from build123d import *

# Parameters (mm, degrees)
BOSS_EXTRUDE1_DEPTH = 5
CUT_EXTRUDE1_DEPTH  = 86.941840799
BOSS_EXTRUDE2_DEPTH = 5
SKETCH7_R           = 4.1
CUT_EXTRUDE2_DEPTH  = 86.941840799
FILLET1_R           = 1


with BuildPart() as part:
    # Sketch1 → Boss-Extrude1 (new body)
    with BuildSketch(Plane(origin=(0, 0, 0), x_dir=(0, 0, -1), z_dir=(1, 0, 0))):
        Polygon((0, 0), (0, -81), (14.142135624, -66.857864376), (28.284271247, -81), (28.284271247, 0), (14.142135624, -14.142135624), align=None)
    extrude(amount=BOSS_EXTRUDE1_DEPTH)

    # Sketch2 → Cut-Extrude1 (cut, through all)
    with BuildSketch(Plane(origin=(5, 0, 0), x_dir=(0, 0, -1), z_dir=(1, 0, 0))):
        Polygon((4, -71.343145751), (12.142135624, -63.201010127), (12.142135624, -17.798989873), (4, -9.656854249), align=None)
        Polygon((16.142135624, -17.798989873), (16.142135624, -63.201010127), (24.284271247, -71.343145751), (24.284271247, -9.656854249), align=None)
    extrude(amount=-CUT_EXTRUDE1_DEPTH, mode=Mode.SUBTRACT)

    # Sketch6 → Boss-Extrude2 (add, through all)
    with BuildSketch(Plane(origin=(5, 0, 0), x_dir=(0, 0, -1), z_dir=(1, 0, 0))):
        with BuildLine():
            Line((20.850339556, -42.5), (16.142135624, -42.5))
            Line((16.142135624, -42.5), (16.142135624, -47.208203932))
            ThreePointArc((16.142135624, -47.208203932), (19.091883092, -45.449747468), (20.850339556, -42.5))
        make_face()
        with BuildLine():
            Line((20.850339556, -38.5), (16.142135624, -38.5))
            Line((16.142135624, -38.5), (16.142135624, -42.5))
            Line((16.142135624, -42.5), (20.850339556, -42.5))
            ThreePointArc((20.850339556, -42.5), (21.068802482, -41.510587075), (21.142135624, -40.5))
            ThreePointArc((21.142135624, -40.5), (21.068802482, -39.489412925), (20.850339556, -38.5))
        make_face()
        with BuildLine():
            Line((16.142135624, -33.791796068), (16.142135624, -38.5))
            Line((16.142135624, -38.5), (20.850339556, -38.5))
            ThreePointArc((20.850339556, -38.5), (19.091883092, -35.550252532), (16.142135624, -33.791796068))
        make_face()
        with BuildLine():
            ThreePointArc((12.142135624, -33.791796068), (9.192388155, -35.550252532), (7.433931691, -38.5))
            Line((7.433931691, -38.5), (12.142135624, -38.5))
            Line((12.142135624, -38.5), (12.142135624, -33.791796068))
        make_face()
        with BuildLine():
            Line((12.142135624, -42.5), (7.433931691, -42.5))
            ThreePointArc((7.433931691, -42.5), (9.192388155, -45.449747468), (12.142135624, -47.208203932))
            Line((12.142135624, -47.208203932), (12.142135624, -42.5))
        make_face()
        with BuildLine():
            Line((12.142135624, -38.5), (7.433931691, -38.5))
            ThreePointArc((7.433931691, -38.5), (7.142135624, -40.5), (7.433931691, -42.5))
            Line((7.433931691, -42.5), (12.142135624, -42.5))
            Line((12.142135624, -42.5), (12.142135624, -38.5))
        make_face()
        with BuildLine():
            Line((7.433931691, -38.5), (4, -38.5))
            Line((4, -38.5), (4, -42.5))
            Line((4, -42.5), (7.433931691, -42.5))
            ThreePointArc((7.433931691, -42.5), (7.142135624, -40.5), (7.433931691, -38.5))
        make_face()
        with BuildLine():
            Line((24.284271247, -38.5), (20.850339556, -38.5))
            ThreePointArc((20.850339556, -38.5), (21.068802482, -39.489412925), (21.142135624, -40.5))
            ThreePointArc((21.142135624, -40.5), (21.068802482, -41.510587075), (20.850339556, -42.5))
            Line((20.850339556, -42.5), (24.284271247, -42.5))
            Line((24.284271247, -42.5), (24.284271247, -38.5))
        make_face()
    extrude(amount=-BOSS_EXTRUDE2_DEPTH)

    # Sketch7 → Cut-Extrude2 (cut, through all)
    with BuildSketch(Plane(origin=(5, 0, 0), x_dir=(0, 0, -1), z_dir=(1, 0, 0))):
        with Locations((14.142135624, -40.5)):
            Circle(SKETCH7_R)
    extrude(amount=-CUT_EXTRUDE2_DEPTH, mode=Mode.SUBTRACT)

    # Fillet1
    fillet1_edges = [part.edges().sort_by_distance(p)[0] for p in [
        (2.5, 0, 0),
        (2.5, 0, -28.284271247),
        (2.5, -81, -28.284271247),
        (2.5, -81, 0),
        (2.5, -17.798989873, -12.142135624),
        (2.5, -63.201010127, -12.142135624),
        (2.5, -71.343145751, -4),
        (2.5, -9.656854249, -4),
        (2.5, -9.656854249, -24.284271247),
        (2.5, -71.343145751, -24.284271247),
        (2.5, -63.201010127, -16.142135624),
        (2.5, -17.798989873, -16.142135624),
    ]]
    fillet(fillet1_edges, radius=FILLET1_R)


solid = part.part
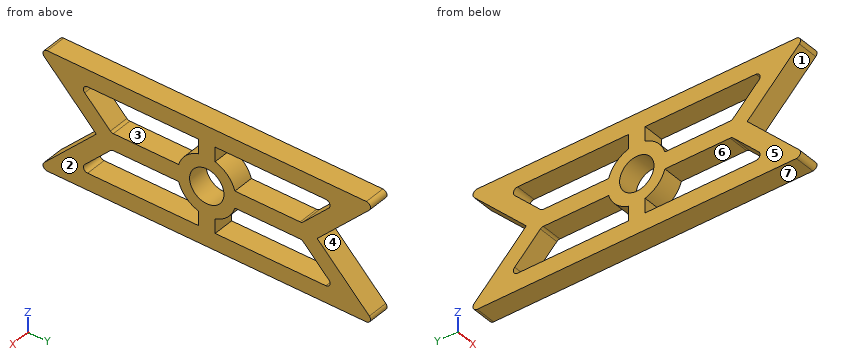
Design review of the part built by this model. Coordinates are the model's own, in mm. Face numbers are marked on the shaded views. A direction names the side the tool comes from. Give positions to 0.01 mm unless a question says otherwise; leave off trailing zeros. Loops run counter-clockwise (first coordinate to the right, second up) from the corner with the lowest first, then second, coordinate; pieces in that order, holes last. Notation, with made-up numbers: (78.25, -3) - (126.25, -3) arc R25 cw to (126.25, 29) - close; hole circle Ø11 at (-39, -14). An arc over 180 degrees is marked (long way). Use CSV: the item, a comma, the result in double quotes. Start each with the question number.
1. Add section B-B (y = -40.5). State the section outline as (x, z) points, plus the area to 3 significant figures.
2. Add section C-C (z = -17.5). State the section outline as (x, y) points.
3. Draft analysis for pull direction Z (two halves, no side actions). For the marked faces 5, 6 and 7, state which applies: released by +Z, released by -Z, zero draft, split by the parting line, or undercut.
4. Machinability: for the marked faces 1, 2, 3 and 4, which of the approach directions +Z, -Z, +X, -X, +Y, -Y give a long, thin tool a straight path to every point of the face, cutting with its end or side? Answer none if there is none.
5. Add section A-A (y = -58). State the section outline as (x, z) points, plus the area to 3 significant figures.
6. Wall thickness on L1, parallel to Z at x = 4.1, y = -26; L2, parallel to Y at x = 1.35, z = -11.5; L3, parallel to Y at x = 1.6, z = -19.5: over which ranges is each line inside the solid? List them lowest first.
7. Insertion check: P1, Ø1.5, axis at x = 2.5, z = -7, coming from the +Y side; P2, Ø2.5, axis at x = 2, z = -5.5, coming from the -Y side; P3, Ø1.7, axis at x = 3.5, z = -6, coming from the +Y side; P4, Ø4, axis at y = -26.5, z = -18.5, coming from the -X side. Each pin has a flat end and moves straight along its axis. Give the tip position at first contact, or say it passes through.
8. Add section D-D (x = 1.55). Count the separate pieces of the cut face and the enclosed holes in it, plus the area to 3 significant figures.
Results found:
1,outline,"(0, -28.28) - (5, -28.28) - (5, -18.24) - (0, -18.24) - close; (0, -10.04) - (5, -10.04) - (5, 0) - (0, 0) - close"
1,area,"100 mm²"
2,outline,"(0, -70.22) - (5, -70.22) - (5, -64.56) - (0, -64.56) - close; (0, -46.64) - (5, -46.64) - (5, -42.85) - (0, -42.85) - close; (0, -38.15) - (5, -38.15) - (5, -34.36) - (0, -34.36) - close; (0, -16.44) - (5, -16.44) - (5, -10.78) - (0, -10.78) - close"
3,face 5,"zero draft"
3,face 6,"undercut"
3,face 7,"released by -Z"
4,face 1,"+X, -X, -Y"
4,face 2,"+Z, -Z, +X, +Y, -Y"
4,face 3,"+X, -X"
4,face 4,"+X, -X, +Y"
5,outline,"(0, -28.28) - (5, -28.28) - (5, -24.28) - (0, -24.28) - close; (0, -16.14) - (5, -16.14) - (5, -12.14) - (0, -12.14) - close; (0, -4) - (5, -4) - (5, 0) - (0, 0) - close"
5,area,"60.0 mm²"
6,L1,"z = -28.28 to -24.28, -16.14 to -12.14, -4 to 0"
6,L2,"y = -69.5 to -63.84, -46.98 to -43.64, -37.36 to -34.02, -17.16 to -11.5"
6,L3,"y = -72.22 to -66.56, -45 to -36, -14.44 to -8.78"
7,P1,"stops at y = -6.25"
7,P2,"stops at y = -76.75"
7,P3,"stops at y = -5.15"
7,P4,"passes through"
8,separate pieces,"1"
8,enclosed holes,"5"
8,area,"1,090 mm²"
